```python
from build123d import *

# Parameters (mm, degrees)
CROQUIS1_R           = 2
BASE_DEPTH           = 1
CROQUIS2_R           = 1.5
CUERPO_DEL_LED_DEPTH = 5.25
CROQUIS3_W           = 0.5
CROQUIS3_H           = 0.5
PINES_DEPTH          = 25.4
CROQUIS4_W           = 0.5
CROQUIS4_H           = 0.5
CORTE_A_CATODO_DEPTH = 1.5
CROQUIS6_W           = 1
CROQUIS6_H           = 4.5
RANURA_DEPTH         = 1
PUNTA_DEL_LED_R      = 1.25


with BuildPart() as part:
    # Croquis1 → Base (new body)
    with BuildSketch(Plane(origin=(0, 0, 0), x_dir=(1, 0, 0), z_dir=(0, 1, 0))):
        with Locations(Location((0, 0, 0), (0, 0, 270))):
            Circle(CROQUIS1_R)
    extrude(amount=BASE_DEPTH)

    # Croquis2 → Cuerpo del LED (add)
    with BuildSketch(Plane(origin=(0, 1, 0), x_dir=(1, 0, 0), z_dir=(0, 1, 0))):
        with Locations(Location((0, 0, 0), (0, 0, 90))):
            Circle(CROQUIS2_R)
    extrude(amount=CUERPO_DEL_LED_DEPTH)

    # Croquis3 → Pines (add)
    with BuildSketch(Plane.XZ):
        with Locations((-1.270142923, 0)):
            Rectangle(CROQUIS3_W, CROQUIS3_H)
        with Locations((1.270172723, 0)):
            Rectangle(CROQUIS3_W, CROQUIS3_H)
    extrude(amount=PINES_DEPTH)

    # Croquis4 → Corte a Catodo (cut)
    with BuildSketch(Plane.XZ.offset(25.4)):
        with Locations((1.270172723, 0)):
            Rectangle(CROQUIS4_W, CROQUIS4_H)
    extrude(amount=-CORTE_A_CATODO_DEPTH, mode=Mode.SUBTRACT)

    # Croquis6 → Ranura (cut)
    with BuildSketch(Plane(origin=(0, 1, 0), x_dir=(1, 0, 0), z_dir=(0, 1, 0))):
        with Locations((2, 0.48044739)):
            Rectangle(CROQUIS6_W, CROQUIS6_H)
    extrude(amount=-RANURA_DEPTH, mode=Mode.SUBTRACT)

    # Punta del Led
    punta_del_led_edges = [part.edges().sort_by_distance(p)[0] for p in [
        (0, 6.25, 1.5),
    ]]
    fillet(punta_del_led_edges, radius=PUNTA_DEL_LED_R)


solid = part.part
```
The model under review builds one solid part; all positions refer to its coordinate system, in mm. A direction names the side the tool comes from. Give positions to 0.01 mm unless a question says otherwise; leave off trailing zeros. Write each loop counter-clockwise with the first axis right and the second up, starting at its lowest first coordinate (ties: lowest second). Pieces come first, ordered by that corner, then holes. Notation, with made-up numbers: M 63,-12 L 94,-12 A19 cw 94,0 Z; hole C 61.5,65 d7. An arc over 180 degrees is marked long. Write item = value, one per line. Start each with the question number.
Q1. For line 1 (X direction, y = -4, z = -0.1); line 2 (Y direction, x = -1.65, z = 0.2); line 3 (Z direction, x = -1.2, y = -16), list the stretches that pass through material, from the lowest coordinate up.
Q2. We need section A-A (y = -6.5). State the section outline as (x, z) points, plus the area to 3 significant figures.
Q3. Machinability: for faces 1 (the face through (-2, 0.49, -0.07)), 2 (the face through (-0.45, 2.97, -1.43)), which of the approach directions +Z, -Z, +X, -X, +Y, -Y give a long, thin tool a straight path to every point of the face, cutting with its end or side? Answer none if there is none.
Q4. Clearance check with a flat-ended pin moving along its axis: pin 1 (0.6 mm diameter, centred on x = -1.5, y = -14.5, fed in from -Z). State where the tip first meets the part, or that it passes through.
Result set:
q1.line_1 = -1.52 to -1.02, 1.02 to 1.52
q1.line_2 = 0 to 1
q1.line_3 = -0.25 to 0.25
q2.outline = M -1.52,-0.25 L -1.02,-0.25 L -1.02,0.25 L -1.52,0.25 Z; M 1.02,-0.25 L 1.52,-0.25 L 1.52,0.25 L 1.02,0.25 Z
q2.area = 0.500 mm2
q3.face_1 = +Y, -Y
q3.face_2 = +Y
q4.pin_1 = -0.25
